Design review of the part shown in the three views and the two pictorial views. Dimensions are in mm from the part's minimum x, y and z. Give positions to 0.01 mm unless a question says otherwise; leave off trailing zeros. Order: outer loops, then holes, each group sorted by start corner. A loop starts at its lowest first (then second) coordinate and runs counter-clockwise, first axis right, second up. Notation, with made-up numbers: (78.5, 46.25) -> (104.5, 46.25) arc R22 ccw to (104.5, 53.25) -> close; hole circle Ø3 at (-30.5, -4.75). An arc over 180 degrees is marked (long way). Use one line per item in the form item = value.
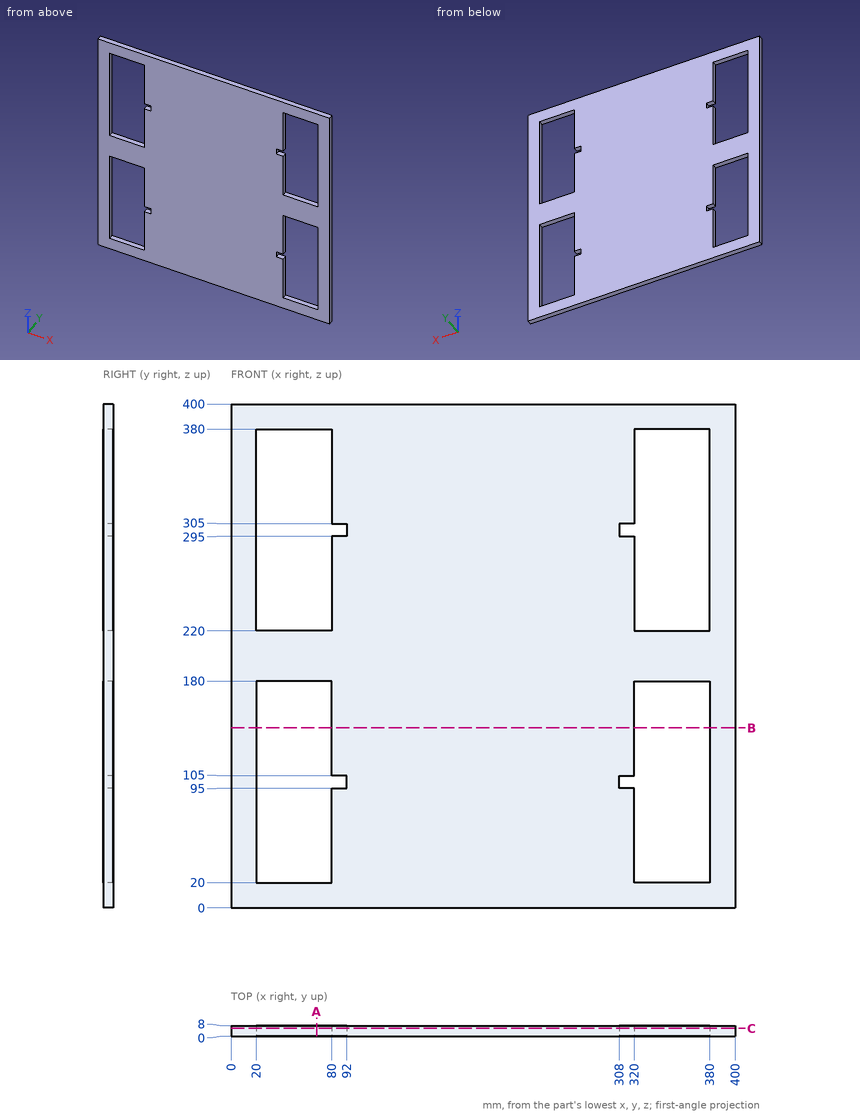
1. Add section B-B on z = 143. Give the boundary of the cut face in (x, y), then the cut area to 3 significant figures.
Values:
outline = (0, 0) -> (20, 0) -> (20, 8) -> (0, 8) -> close; (80, 0) -> (320, 0) -> (320, 8) -> (80, 8) -> close; (380, 0) -> (400, 0) -> (400, 8) -> (380, 8) -> close
area = 2,240 mm^2
2. For L1, parallel to Z at x = 61, y = 6.25; L2, parallel to X at y = 5.25, z = 161; L3, parallel to X at y = 6.75, z = 297.5, list the stretches that pass through material, from the lowest coordinate up.
Values:
L1 = 0 to 20, 180 to 220, 380 to 400
L2 = 0 to 20, 80 to 320, 380 to 400
L3 = 0 to 20, 92 to 308, 380 to 400
3. Add section C-C on y = 6. Count the separate pieces of the cut face and the enclosed holes in it, then the cut area to 3 significant figures.
Values:
separate_pieces = 1
enclosed_holes = 4
area = 121,000 mm^2
4. Add section A-A on x = 68. Give the boundary of the cut face in (y, z).
Values:
outline = (0, 0) -> (8, 0) -> (8, 20) -> (0, 20) -> close; (0, 180) -> (8, 180) -> (8, 220) -> (0, 220) -> close; (0, 380) -> (8, 380) -> (8, 400) -> (0, 400) -> close
5. For pin 1 Ø2.5 at (x, y) = (311.5, 4.5) entering from -Z, flat-tipped, find the tip position at first contact; note if it passes through.
Values:
pin_1 = 0
